Autodesk Inventor part; units mm, degrees
ref_plane "YZ Plane" through (0, 0, 0) normal (1, 0, 0) x (0, 1, 0)
ref_plane "XZ Plane" through (0, 0, 0) normal (0, 1, 0) x (-1, 0, 0)
sketch "Sketch1" plane through (0, 0, 0) normal (0, 0, 1) x (1, 0, 0)
  circle A0 centre (0, 0) radius 0.515
  dimension "d0" = 1.03
extrude "Extrusion1" add sketch "Sketch1" along normal blind 13.5
thread "Thread1"
sketch "Sketch2" plane through (0, 0, 0) normal (1, 0, 0) x (0, 1, 0)
  line L0 (-0.515, 13.5) -> (0.515, 13.5)
  line L1 (-0.515, 0) -> (-0.515, 13.5)
  line L2 (0.515, 0) -> (0.515, 13.5)
  arc A0 (0, 0) -> (0.515, 0.1161) centre (0, 1.2) ccw
  line L3 (-0.515, 0) -> (0.515, 0)
  line L4 (0.515, 0.1161) -> (0.515, 0)
  line L5 (0, 0) -> (0.515, 0)
  line L6 (0, -2.9344) -> (0, 17.4057)
  point P0 (0, 0)
  point P1 (0, 0)
revolve "Revolution1" cut sketch "Sketch2" angle 360 about axis through (0, 0, -10) along (0, 0, 1) contours A0 L2 L3
ref_plane "Work Plane3" through (0, 0, 6.75) normal (0, 0, 1) x (1, 0, 0)
mirror "Mirror1" [suppressed]
ref_plane "Work Plane4" through (0, 0, 13.5) normal (0, 0, 1) x (1, 0, 0)
sketch "Sketch3" plane through (0, 0, 13.5) normal (0, 0, 1) x (1, 0, 0)
  circle A0 centre (0, 0) radius 0.5
  circle A1 centre (0, 0) radius 0.515
  dimension "d12" = 1
extrude "Extrusion2" [suppressed]
sketch "Sketch4" plane through (0, 0, 13.5) normal (0, 0, 1) x (1, 0, 0)
  circle A0 centre (0, 0) radius 0.5
  dimension "d15" = 1
extrude "Extrusion3" add sketch "Sketch4" along normal blind 1
fillet "Fillet1" radius 0.2 1 edges at (-0.5, 0, 14.5)
equation "\"d10\" = 0.5 * d1"
equation "\"d11\" = d1"
properties part number "MU_Motor_Thread_Modified" material "Brass, Soft Yellow"
The listing builds one solid part. Answer for the finished solid, in the listing's coordinates (mm). A direction names the side the tool comes from. Round coordinates to 2 decimals unless told otherwise and drop trailing zeros. Write each loop counter-clockwise with the first axis right and the second up, starting at its lowest first coordinate (ties: lowest second). Pieces come first, ordered by that corner, then holes. Notation, with made-up numbers: (-19.5, 71.5) - (23.5, 71.5) arc R14 ccw to (23.5, 85.5) - close; hole circle Ø4 at (-10.5, 58). An arc over 180 degrees is marked (long way). Use a Markdown table: item, result. Add a question column.
1. Consider line 1 (X direction, y = 0.05, z = 13.75); line 2 (Y direction, x = 0.05, z = 5.25); line 3 (Z direction, x = 0, y = 0.05). Determine where each line is inside the solid, lowest interval first.
2. A tool of negligible diameter and unlimited length cuts with its end or side. For faces 1 (the face through (-0.41, 0.31, 6.71)), 2 (the face through (-0.108, 0.488, 13.894)), from which of +Z, -Z, +X, -X, +Y, -Y can it reach the whole face along a straight path? Write none if from no direction.
3. The part is cut by section A-A (z = 3). Write down the section's boundary in (x, y) (3 decimals), and give its area (3 significant figures).
Reported:
| question | item | result |
|---|---|---|
| 1 | line 1 | -0.5 to 0.5 |
| 1 | line 2 | -0.51 to 0.51 |
| 1 | line 3 | 0 to 14.5 |
| 2 | face 1 | +Z, -Z |
| 2 | face 2 | +Z |
| 3 | outline | circle Ø1.03 at (0, 0) |
| 3 | area | 0.833 mm^2 |
